```python
from build123d import *

# Parameters (mm, degrees)
SKETCH1_W           = 56
SKETCH1_H           = 56
BOSS_EXTRUDE1_DEPTH = 1.3
SKETCH2_W           = 6.175
SKETCH2_H           = 17
BOSS_EXTRUDE2_DEPTH = 7.5
SKETCH3_W           = 12.35
SKETCH3_H           = 17
BOSS_EXTRUDE3_DEPTH = 7.5
BOSS_EXTRUDE4_DEPTH = 1.5
SKETCH5_W           = 56
SKETCH5_H           = 56
BOSS_EXTRUDE5_DEPTH = 1.3
SKETCH7_R           = 2.5
CUT_EXTRUDE1_DEPTH  = 1.3
SKETCH8_W           = 6.175
SKETCH8_H           = 8.5
BOSS_EXTRUDE6_DEPTH = 15


with BuildPart() as part:
    # Sketch1 → Boss-Extrude1 (new body)
    with BuildSketch(Plane.XY):
        with Locations((28, 28)):
            Rectangle(SKETCH1_W, SKETCH1_H)
    extrude(amount=BOSS_EXTRUDE1_DEPTH)

    # Sketch2 → Boss-Extrude2 (add)
    with BuildSketch(Plane.XY.offset(1.3)):
        Polygon((14, 28), (14, 41.65), (0.1, 41.65), (0.1, 14.35), (14, 14.35), align=None)
        Polygon((27.9, 41.65), (14, 41.65), (14, 28), (14, 14.35), (27.9, 14.35), align=None)
        with Locations((38.9125, 37)):
            Rectangle(SKETCH2_W, SKETCH2_H)
        with Locations((45.0875, 37)):
            Rectangle(SKETCH2_W, SKETCH2_H)
        with Locations((45.0875, 19)):
            Rectangle(SKETCH2_W, SKETCH2_H)
        with Locations((38.9125, 19)):
            Rectangle(SKETCH2_W, SKETCH2_H)
    extrude(amount=BOSS_EXTRUDE2_DEPTH)

    # Sketch3 → Boss-Extrude3 (add)
    with BuildSketch(Plane.XY.offset(8.8)):
        with Locations((42, 37)):
            Rectangle(SKETCH3_W, SKETCH3_H)
        with Locations((42, 19)):
            Rectangle(SKETCH3_W, SKETCH3_H)
    extrude(amount=BOSS_EXTRUDE3_DEPTH)

    # Sketch4 → Boss-Extrude4 (add)
    with BuildSketch(Plane.XY.offset(8.8)):
        Polygon((26.5, 23.35), (14, 23.35), (1.5, 23.35), (1.5, 36.35), (26.5, 36.35), align=None)
    extrude(amount=BOSS_EXTRUDE4_DEPTH)

    # Sketch5 → Boss-Extrude5 (add)
    with BuildSketch(Plane.XY.offset(1.3)):
        with Locations((-28, 28)):
            Rectangle(SKETCH5_W, SKETCH5_H)
    extrude(amount=-BOSS_EXTRUDE5_DEPTH)

    # Sketch7 → Cut-Extrude1 (cut)
    with BuildSketch(Plane.XY.offset(1.3)):
        with Locations((-52, 52)):
            Circle(SKETCH7_R)
        with Locations((-52, 4)):
            Circle(SKETCH7_R)
        with Locations((52, 4)):
            Circle(SKETCH7_R)
        with Locations((52, 52)):
            Circle(SKETCH7_R)
    extrude(amount=-CUT_EXTRUDE1_DEPTH, mode=Mode.SUBTRACT)

    # Sketch8 → Boss-Extrude6 (add)
    with BuildSketch(Plane.XY.offset(1.3)):
        Polygon((-7.825, 36.5), (-14, 36.5), (-14, 28), (-14, 19.5), (-7.825, 19.5), align=None)
        with Locations((-17.0875, 32.25)):
            Rectangle(SKETCH8_W, SKETCH8_H)
        with Locations((-17.0875, 23.75)):
            Rectangle(SKETCH8_W, SKETCH8_H)
    extrude(amount=BOSS_EXTRUDE6_DEPTH)


solid = part.part
```
Verification items for the finished model (mm, model axes). A direction names the side the tool comes from. Give positions to 0.01 mm unless a question says otherwise; leave off trailing zeros. Order: outer loops, then holes, each group sorted by start corner. A loop starts at its lowest first (then second) coordinate and runs counter-clockwise, first axis right, second up. Notation, with made-up numbers: M 18,31.25 L 28,31.25 A27 ccw 28,47.25 Z; hole C -25,68 d4. An arc over 180 degrees is marked long. Return JSON: item names as keys, results as strings. Group by question number.
1) Section check A-A on x = -52. Record the cut outline in (y, z).
2) Go/stop test with flat-tipped pins: pin 1 Ø8 at (x, z) = (-3.5, 5.5) entering from -Y; pin 2 Ø6 at (y, z) = (27.5, 5.5) entering from +X (3 decimals); pin 3 Ø8.5 at (x, z) = (15.5, 4.5) entering from +Y; pin 4 Ø1 at (x, z) = (-8.5, 6) entering from +Y. Record where each tip stops, or that it passes through.
3) Mould release check, pull along Y, two halves, no side actions. Record for faces 1 (the face through (-49.69, 3.04, 0.66)), 2 (the face through (-14, 36.5, 9)), 3 (the face through (-7.825, 28, 9)): pulls with the +Y half, pulls with the -Y half, needs draft (parallel to the pull), parting line crosses it, or undercut.
4) Access from +Z, -Z, +X, -X, +Y, -Y to the whole of each face (thin tool, end or side, straight path). Record for faces 4 (the face through (42, 10.5, 9)), 5 (the face through (27.9, 28, 5)), 6 (the face through (42, 27.5, 9)).
5) Scan lines: line 1 (Y direction, x = -52, z = 0.3); line 2 (X direction, y = 28, z = 8.25) (3 decimals); line 3 (Y direction, x = 45, z = 8.25). Record each from-to range of solid material in increasing order.
6) Section check D-D on x = -10. Record the cut outline in (y, z), and give its area (3 significant figures).
7) Section check C-C on y = 30. Record the cut outline in (x, z) (3 decimals), and give its area (3 significant figures).
8) Section check B-B on y = 52. Record the cut outline in (x, z), and give its area (3 significant figures).
Answer block:
{
 "1": {"outline": "M 0,0 L 1.5,0 L 1.5,1.3 L 0,1.3 Z; M 6.5,0 L 49.5,0 L 49.5,1.3 L 6.5,1.3 Z; M 54.5,0 L 56,0 L 56,1.3 L 54.5,1.3 Z"},
 "2": {"pin 1": "stops at y = 14.35", "pin 2": "stops at x = 48.175", "pin 3": "stops at y = 56", "pin 4": "stops at y = 36.5"},
 "3": {"face 1": "undercut", "face 2": "pulls with the +Y half", "face 3": "needs draft"},
 "4": {"face 4": "+Z, +X, -X, -Y", "face 5": "+Z, +Y, -Y", "face 6": "+Z, +X"},
 "5": {"line 1": "y = 0 to 1.5, 6.5 to 49.5, 54.5 to 56", "line 2": "x = -20.175 to -7.825, 0.1 to 27.9", "line 3": "y = 10.5 to 27.5, 28.5 to 45.5"},
 "6": {"outline": "M 0,0 L 56,0 L 56,1.3 L 36.5,1.3 L 36.5,16.3 L 19.5,16.3 L 19.5,1.3 L 0,1.3 Z", "area": "328 mm^2"},
 "7": {"outline": "M -56,0 L 56,0 L 56,1.3 L 48.175,1.3 L 48.175,16.3 L 35.825,16.3 L 35.825,1.3 L 27.9,1.3 L 27.9,8.8 L 26.5,8.8 L 26.5,10.3 L 1.5,10.3 L 1.5,8.8 L 0.1,8.8 L 0.1,1.3 L -7.825,1.3 L -7.825,16.3 L -20.175,16.3 L -20.175,1.3 L -56,1.3 Z", "area": "762 mm^2"},
 "8": {"outline": "M -56,0 L -54.5,0 L -54.5,1.3 L -56,1.3 Z; M -49.5,0 L 49.5,0 L 49.5,1.3 L -49.5,1.3 Z; M 54.5,0 L 56,0 L 56,1.3 L 54.5,1.3 Z", "area": "133 mm^2"}
}
